```python
from build123d import *

# Parameters (mm, degrees)
SKETCH_1_W          = 50
SKETCH_1_H          = 65.5
EXTRUDE_1_DEPTH     = 5
SKETCH_4_W          = 10
SKETCH_4_H          = 65.5
EXTRUDE_2_DEPTH     = 70
CUT_EXTRUDE_1_DEPTH = 5
FILLET_7_R          = 5


with BuildPart() as part:
    # 스케치1 → 보스-돌출1 (new body)
    with BuildSketch(Plane.XY):
        Rectangle(SKETCH_1_W, SKETCH_1_H)
    extrude(amount=EXTRUDE_1_DEPTH)

    # 스케치4 → 보스-돌출2 (add)
    with BuildSketch(Plane.XY.offset(5)):
        with Locations((-20, 0)):
            Rectangle(SKETCH_4_W, SKETCH_4_H)
    extrude(amount=EXTRUDE_2_DEPTH)

    # 스케치2 → 컷-돌출1 (cut)
    with BuildSketch(Plane.XY.offset(5)):
        with BuildLine():
            Line((-10, -28.2), (20, -28.2))
            ThreePointArc((20, -28.2), (23.2, -25), (20, -21.8))
            Line((20, -21.8), (-10, -21.8))
            ThreePointArc((-10, -21.8), (-13.2, -25), (-10, -28.2))
        make_face()
        with BuildLine():
            Line((-10, -3.2), (20, -3.2))
            ThreePointArc((20, -3.2), (23.2, 0), (20, 3.2))
            Line((20, 3.2), (-10, 3.2))
            ThreePointArc((-10, 3.2), (-13.2, 0), (-10, -3.2))
        make_face()
        with BuildLine():
            Line((-10, 21.8), (20, 21.8))
            ThreePointArc((20, 21.8), (23.2, 25), (20, 28.2))
            Line((20, 28.2), (-10, 28.2))
            ThreePointArc((-10, 28.2), (-13.2, 25), (-10, 21.8))
        make_face()
    extrude(amount=-CUT_EXTRUDE_1_DEPTH, mode=Mode.SUBTRACT)

    # 필렛7
    # the kernel refuses this fillet: 5 mm, written as the material it adds along each edge
    with BuildSketch(Plane(origin=(-15, -32.75, 5), x_dir=(0, 0, 1), z_dir=(0, 1, 0))) as fillet_7_piece_1_section:
        with BuildLine():
            CenterArc((FILLET_7_R, FILLET_7_R), FILLET_7_R, 180, 90)
            Line((0, FILLET_7_R), (0, 0))
            Line((0, 0), (FILLET_7_R, 0))
        make_face()
    fillet_7_piece_1 = extrude(amount=65.5, mode=Mode.PRIVATE)
    fillet_7_piece_1 = fillet_7_piece_1 - Plane(origin=(-10, -25, 6.131975571), x_dir=(0, 1, 0), z_dir=(0, 0, 1)) * Cylinder(3.2, 151, mode=Mode.PRIVATE)
    fillet_7_piece_1 = fillet_7_piece_1 - Plane(origin=(-10, 0, 6.131975571), x_dir=(0, 1, 0), z_dir=(0, 0, 1)) * Cylinder(3.2, 151, mode=Mode.PRIVATE)
    fillet_7_piece_1 = fillet_7_piece_1 - Plane(origin=(-10, 25, 6.131975571), x_dir=(0, 1, 0), z_dir=(0, 0, 1)) * Cylinder(3.2, 151, mode=Mode.PRIVATE)
    add(fillet_7_piece_1)


solid = part.part
```
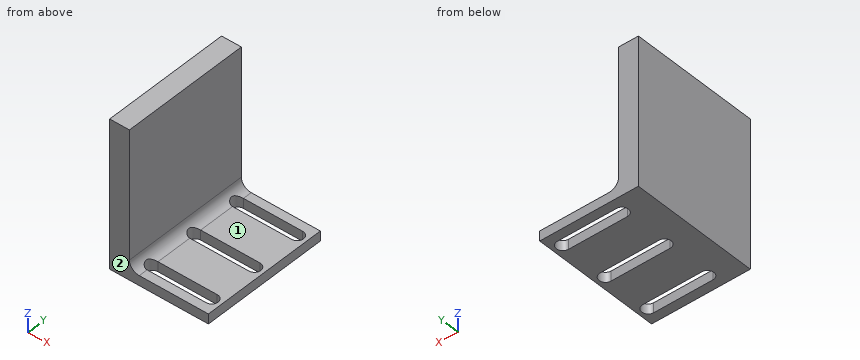
Check sheet for the modelled part. Datum: model origin and axes. Units: mm. Face numbers are marked on the shaded views. A direction names the side the tool comes from. Round coordinates to 2 decimals unless told otherwise and drop trailing zeros. Order: outer loops, then holes, each group sorted by start corner. A loop starts at its lowest first (then second) coordinate and runs counter-clockwise, first axis right, second up. Notation, with made-up numbers: (35, -32) -> (76, -32) arc R19 cw to (76, -9) -> close; hole circle Ø8 at (66.5, -6.75). An arc over 180 degrees is marked (long way). One line per item, written item: value. Start each with the question number.
Q1. Thickness scan on line 1 (X direction, y = 19, z = 45); line 2 (Z direction, x = 12, y = 20). Record the ranges inside material, lowest first.
Q2. Set-up check for the marked faces 1 and 2: record each of +Z, -Z, +X, -X, +Y, -Y from which the full face is reachable in a straight line by a thin tool's end or side.
Q3. Gauge pin test, flat ends, axial feed: pin 1 Ø10 at (y, z) = (9.5, 45) entering from +X; pin 2 Ø10.5 at (x, y) = (11.5, -11) entering from +Z; pin 3 Ø10 at (x, z) = (-9.5, 64) entering from +Y; pin 4 Ø12 at (x, y) = (13, 22) entering from -Z. Record the tip position at first contact, or that the pin passes through.
Q4. Cross-section at B-B (x = -7). Record the boundary of the cut face in (y, z).
Q5. Cross-section at C-C (y = 14.5). Record the boundary of the cut face in (x, z), and give its area (3 significant figures).
Q6. Cross-section at D-D (z = 48.5). Record the boundary of the cut face in (x, y), and give its area (3 significant figures).
Q7. Cross-section at A-A (y = 25). Record the boundary of the cut face in (x, z).
Completed:
1. line 1: x = -25 to -15
1. line 2: z = 0 to 5
2. face 1: +Z, +X, +Y, -Y
2. face 2: +Z, -Z, +X, -X, -Y
3. pin 1: stops at x = -15
3. pin 2: stops at z = 5
3. pin 3: passes through
3. pin 4: stops at z = 0
4. outline: (-32.75, 0) -> (-28.2, 0) -> (-28.2, 5) -> (-32.75, 5) -> close; (-21.8, 0) -> (-3.2, 0) -> (-3.2, 5) -> (-21.8, 5) -> close; (3.2, 0) -> (21.8, 0) -> (21.8, 5) -> (3.2, 5) -> close; (28.2, 0) -> (32.75, 0) -> (32.75, 5) -> (28.2, 5) -> close
5. outline: (-25, 0) -> (25, 0) -> (25, 5) -> (-10, 5) arc R5 cw to (-15, 10) -> (-15, 75) -> (-25, 75) -> close
5. area: 955 mm²
6. outline: (-25, -32.75) -> (-15, -32.75) -> (-15, 32.75) -> (-25, 32.75) -> close
6. area: 655 mm²
7. outline: (-25, 0) -> (-13.2, 0) -> (-13.2, 6.16) arc R5 cw to (-15, 10) -> (-15, 75) -> (-25, 75) -> close; (23.2, 0) -> (25, 0) -> (25, 5) -> (23.2, 5) -> close
